Solid Edge part; units mm, degrees
sketch "Sketch1" plane through (0, 0, 0) normal (0, -1, 0) x (1, 0, 0)
  line L0 (-99.3424, -56.6999) -> (-81.7165, -56.6999)
  line L1 (-81.7165, -56.6999) -> (-81.7165, -60.9006)
  line L2 (-84.199, -60.9006) -> (-81.7165, -60.9006)
  line L3 (-84.199, -58.3606) -> (-84.199, -60.9006)
  line L4 (-94.8512, -58.3606) -> (-84.199, -58.3606)
  line L5 (-94.8512, -69.321) -> (-94.8512, -58.3606)
  line L6 (-89.3922, -74.78) -> (-94.8512, -69.321)
  line L7 (-89.3922, -74.78) -> (-94.8522, -80.24)
  line L8 (-94.8522, -80.24) -> (-99.3424, -75.7499)
  line L9 (-99.3424, -75.7499) -> (-99.3424, -56.6999)
revolve "RevolvedProtrusion1" add sketch "Sketch1" angle 360 about axis through (-23.4251, 0, -63.5843) along (0, 0, 1)
chamfer "Chamfer_1" distance 6.35 angle 30 1 edges at (52.4921, 0, -56.6999) measured on face at (28.7048, 49.0932, -56.6999)
chamfer "Chamfer_2" distance 2.54 angle 30 1 edges at (34.8663, 0, -56.6999) measured on face at (24.3444, 44.9869, -56.6999)
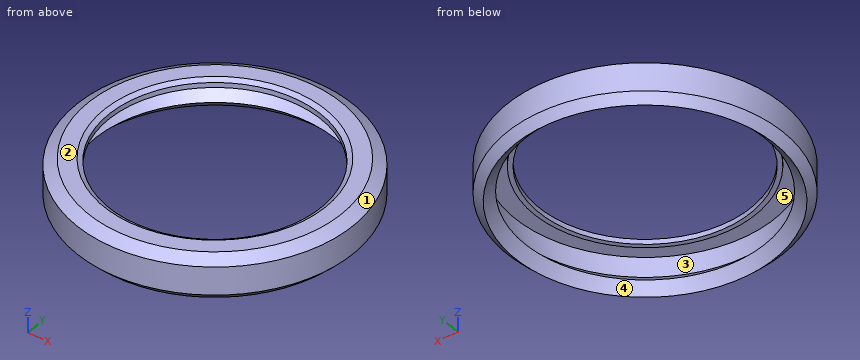
Read the model definition and answer for the solid it produces. Units are mm, in the model's axes. Face numbers are marked on the shaded views. A direction names the side the tool comes from. Round coordinates to 2 decimals unless told otherwise and drop trailing zeros. Loops run counter-clockwise (first coordinate to the right, second up) from the corner with the lowest first, then second, coordinate; pieces in that order, holes last.
Q1. Section B-B on y = 0 is taken. Write down the section's boundary in (x, z).
Q2. Each of these flat-tipped pins is pushed along its axis until it touches: pin 1 (5 mm diameter, centred on x = -11.5, z = -73, fed in from +Y); pin 2 (10 mm diameter, centred on y = 37.5, z = -63.5, fed in from -X); pin 3 (10 mm diameter, centred on y = -9, z = -76.5, fed in from -X). Where does it stop, or does it pass through?
Q3. Which of the six approach directions +Z, -Z, +X, -X, +Y, -Y give full straight-line access (tool end or side, diameter ignored) to the marked faces 4 and 5?
Q4. Section A-A on z = -66 is taken. Write down the section's boundary in (x, y).
Q5. Determine the mould class of the marked faces 1, 2 and 3 for opening direction X: released by +X, released by -X, zero draft, split by the parting line, or undercut.
Q6. Consider probe 1 along X at (y, z) = (-7.5, -59.5); probe 2 along Y at (x, z) = (-76.5, -59); probe 3 along Y at (x, z) = (-46, -58.5). Determine where each line is inside the solid, lowest interval first.
Output:
1. outline: (-99.34, -75.75) - (-94.85, -80.24) - (-89.39, -74.78) - (-94.85, -69.32) - (-94.85, -58.36) - (-84.2, -58.36) - (-84.2, -60.9) - (-81.72, -60.9) - (-81.72, -58.17) - (-84.26, -56.7) - (-92.99, -56.7) - (-99.34, -60.37) - close; (34.87, -60.9) - (37.35, -60.9) - (37.35, -58.36) - (48, -58.36) - (48, -69.32) - (42.54, -74.78) - (48, -80.24) - (52.49, -75.75) - (52.49, -60.37) - (46.14, -56.7) - (37.41, -56.7) - (34.87, -58.17) - close
2. pin 1: stops at y = 75.33
2. pin 2: stops at x = -92.03
2. pin 3: stops at x = -99.23
3. face 4: -Z
3. face 5: none
4. outline: circle Ø151.83 at (-23.43, 0); hole circle Ø142.85 at (-23.43, 0)
5. face 1: split by the parting line
5. face 2: zero draft
5. face 3: undercut
6. probe 1: x = -97.46 to -94.46, -83.73 to -81.23, 34.38 to 36.88, 47.61 to 50.61
6. probe 2: y = -50.92 to -47.8, -29.61 to -24.1, 24.1 to 29.61, 47.8 to 50.92
6. probe 3: y = -69.09 to -67.76, -56.43 to -53.74, 53.74 to 56.43, 67.76 to 69.09
